The listing builds one solid part. Answer for the finished solid, in the listing's coordinates (mm). A direction names the side the tool comes from. Give positions to 0.01 mm unless a question says otherwise; leave off trailing zeros. Order: outer loops, then holes, each group sorted by start corner. A loop starts at its lowest first (then second) coordinate and runs counter-clockwise, first axis right, second up. Notation, with made-up numbers: (-8, -16) - (7, -16) arc R30 ccw to (7, 20) - close; hole circle Ø9 at (41.5, -1). An arc over 180 degrees is marked (long way). Use a Markdown table: item, result. Add a question column.
1) The mould has two halves that part along Y. Classify faces 5 (the face through (-16.926, 7, 5)), 6 (the face through (-26, -2, 29)), 7 (the face through (-13.66, -9.32, 5.2)), 8 (the face through (-32, 5, 5)): released by +Y, released by -Y, zero draft, split by the parting line, or undercut.
2) Straight lines are drawn through the part: line 1 (Z direction, x = -22.75, y = 5.5); line 2 (Y direction, x = -22, z = 15); line 3 (Y direction, x = -16.25, z = 26). For each, find the intervals that lie inside material, in ascending order.
3) Flat-ended cylindrical pins translate along their axes: pin 1 (1.5 mm diameter, centred on x = -17, z = 13.5, fed in from -Y); pin 2 (3.5 mm diameter, centred on x = -22.93, z = 9.99, fed in from -Y); pin 3 (12 mm diameter, centred on x = -14.5, z = 34.5, fed in from +Y). Find the tip coordinate at first contact, or state that the pin passes through.
4) For faces 1 (the face through (-16.926, -5, 17)), 2 (the face through (-30.926, -5, 21)), 3 (the face through (-16.926, -17, 5)), 4 (the face through (-23, -1, 20.744)), determine the directions among +Z, -Z, +X, -X, +Y, -Y from which every point of the face is accessible in a straight line to the end or side of a thin tool.
5) Find section D-D, the plane x = -19. Determine the outline of the cut face in (y, z).
6) Find section B-B, the plane x = -13. Determine the outline of the cut face in (y, z), plus the area to 3 significant figures.
7) Find section A-A, the plane y = 4.3. Determine the outline of the cut face in (x, z), plus the area to 3 significant figures.
8) Find section C-C, the plane y = -17. Determine the outline of the cut face in (x, z), plus the area to 3 significant figures.
from build123d import *

# Parameters (mm, degrees)
F0_R          = 1.3
F1_DEPTH      = 2
F2_W          = 12
F2_H          = 3
F3_DEPTH      = 18
F3_DEPTH_BACK = 12
F4_W          = 5
F4_H          = 3
F4_W_2        = 2
F4_H_2        = 35.8160760757
F5_DEPTH      = 2
F6_W          = 2
F6_H          = 35.8160760757
F7_DEPTH      = 2
F9_DEPTH      = 5
F11_DEPTH     = 5
F12_R         = 1
F13_DEPTH     = 5
F14_W         = 2.25
F14_H         = 11.5
F15_DEPTH     = 3
F16_R         = 1.2
F17_DEPTH     = 3
F19_DEPTH     = 2


with BuildPart() as f1:
    # F0 (on Front) → F1 (new body)
    with BuildSketch(Plane.XZ):
        with BuildLine():
            Line((-16.9256870747, 6.6775220651), (-16.9256870747, 9.9935981408))
            Line((-16.9256870747, 9.9935981408), (-16.9256870747, 10.6775220651))
            Line((-16.9256870747, 10.6775220651), (-16.9256870747, 42.4935981408))
            ThreePointArc((-16.9256870747, 42.4935981408), (-22.9256870747, 48.4935981408), (-28.9256870747, 42.4935981408))
            Line((-28.9256870747, 42.4935981408), (-28.9256870747, 9.9935981408))
            Line((-28.9256870747, 9.9935981408), (-28.9256870747, 6.6775220651))
            Line((-28.9256870747, 6.6775220651), (-16.9424954802, 6.6775220651))
            Line((-16.9424954802, 6.6775220651), (-16.9256870747, 6.6775220651))
        make_face()
        with Locations((-22.9256870747, 9.9935981408)):
            Circle(F0_R, mode=Mode.SUBTRACT)
        with Locations((-22.9256870747, 42.4935981408)):
            Circle(F0_R, mode=Mode.SUBTRACT)
    extrude(amount=F1_DEPTH)

    # F2 (on face) → F3 (join, two sides)
    with BuildSketch(Plane.XZ.offset(2)) as f3_sk:
        with Locations((-22.9256870747, 5.1775220651)):
            Rectangle(F2_W, F2_H)
    extrude(amount=F3_DEPTH)
    extrude(f3_sk.sketch, amount=-F3_DEPTH_BACK)

    # F4 (on face) → F5 (join)
    with BuildSketch(Plane.YZ.offset(-16.9256870747)):
        Polygon((-13, 6.6775220651), (-2, 6.6775220651), (-2, 42.4935981408), align=None)
        Polygon((0, 3.6775220651), (0, 6.6775220651), (-2, 6.6775220651), (-13, 6.6775220651), (-13, 3.6775220651), align=None)
        with Locations((2.5, 5.1775220651)):
            Rectangle(F4_W, F4_H)
        with Locations((-1, 24.5855601029)):
            Rectangle(F4_W_2, F4_H_2)
    extrude(amount=F5_DEPTH)

    # F6 (on face) → F7 (join)
    with BuildSketch(Plane(origin=(-28.9256870747, 0, 0), x_dir=(0, -1, 0), z_dir=(-1, 0, 0))):
        Polygon((0, 6.6775220651), (-5, 6.6775220651), (-5, 3.6775220651), (13, 3.6775220651), (13, 6.6775220651), (2, 6.6775220651), align=None)
        Polygon((2, 42.4935981408), (2, 6.6775220651), (13, 6.6775220651), align=None)
        with Locations((1, 24.5855601029)):
            Rectangle(F6_W, F6_H)
    extrude(amount=F7_DEPTH)

    # F8 (on face) → F9 (join)
    with BuildSketch(Plane(origin=(-30.9256870747, 0, 0), x_dir=(0, -1, 0), z_dir=(-1, 0, 0))):
        Polygon((0, 6.6775220651), (-5, 6.6775220651), (-5, 3.6775220651), (13, 3.6775220651), (13, 6.6775220651), align=None)
    extrude(amount=F9_DEPTH)

    # F10 (on face) → F11 (join)
    with BuildSketch(Plane.YZ.offset(-14.9256870747)):
        Polygon((0, 6.6775220651), (-13, 6.6775220651), (-13, 3.6775220651), (5, 3.6775220651), (5, 6.6775220651), align=None)
    extrude(amount=F11_DEPTH)

    # F12 (on face) → F13 (cut)
    with BuildSketch(Plane.XY.offset(6.6775220651)):
        with Locations((-32.9256870747, 2)):
            Circle(F12_R)
        with Locations((-12.9256870747, 2)):
            Circle(F12_R)
        with Locations((-12.9256870747, -10)):
            Circle(F12_R)
        with Locations((-22.9256870747, -5)):
            Circle(F12_R)
        with Locations((-32.9256870747, -10)):
            Circle(F12_R)
        with Locations((-22.9256870747, -17)):
            Circle(F12_R)
    extrude(amount=-F13_DEPTH, mode=Mode.SUBTRACT)

    # F14 (on face) → F15 (cut)
    with BuildSketch(Plane(origin=(0, 0, 0), x_dir=(-1, 0, 0), z_dir=(0, 1, 0))):
        with Locations((24.0506870747, 26.4935981408)):
            Rectangle(F14_W, F14_H)
        with Locations((21.8006870747, 26.4935981408)):
            Rectangle(F14_W, F14_H)
    extrude(amount=-F15_DEPTH, mode=Mode.SUBTRACT)

    # F16 (on face) → F17 (cut)
    with BuildSketch(Plane.XY.offset(6.6775220651)):
        with Locations((-18.7256870747, 4.3)):
            Circle(F16_R)
    extrude(amount=-F17_DEPTH, mode=Mode.SUBTRACT)

    # F18 (on face) → F19 (join)
    with BuildSketch(Plane(origin=(0, 0, 0), x_dir=(-1, 0, 0), z_dir=(0, 1, 0))):
        with BuildLine():
            Line((28.9256870747, 42.4935981408), (30.9256870747, 42.4935981408))
            ThreePointArc((30.9256870747, 42.4935981408), (22.9256870747, 50.4935981408), (14.9256870747, 42.4935981408))
            Line((14.9256870747, 42.4935981408), (16.9256870747, 42.4935981408))
            ThreePointArc((16.9256870747, 42.4935981408), (22.9256870747, 48.4935981408), (28.9256870747, 42.4935981408))
        make_face()
    extrude(amount=-F19_DEPTH)


solid = f1.part
The answers:
| question | item | result |
|---|---|---|
| 1 | face 5 | zero draft |
| 1 | face 6 | released by -Y |
| 1 | face 7 | undercut |
| 1 | face 8 | released by +Y |
| 2 | line 1 | 3.68 to 6.68 |
| 2 | line 2 | -2 to 0 |
| 2 | line 3 | -7.07 to 0 |
| 3 | pin 1 | y = -11.13 |
| 3 | pin 2 | y = -2 |
| 3 | pin 3 | y = 0 |
| 4 | face 1 | +Z, -Y |
| 4 | face 2 | +Z, -X, +Y, -Y |
| 4 | face 3 | +Z, -Z, +X, -Y |
| 4 | face 4 | +Y, -Y |
| 5 | outline | (-20, 3.68) - (3.13, 3.68) - (3.13, 6.68) - (0, 6.68) - (0, 49.46) - (-2, 49.46) - (-2, 6.68) - (-20, 6.68) - close; (5.47, 3.68) - (10, 3.68) - (10, 6.68) - (5.47, 6.68) - close |
| 6 | outline | (-13, 3.68) - (-11, 3.68) - (-11, 6.68) - (-13, 6.68) - close; (-9, 3.68) - (1, 3.68) - (1, 6.68) - (-9, 6.68) - close; (3, 3.68) - (5, 3.68) - (5, 6.68) - (3, 6.68) - close |
| 6 | area | 42.0 mm2 |
| 7 | outline | (-35.93, 3.68) - (-19.93, 3.68) - (-19.93, 6.68) - (-35.93, 6.68) - close; (-17.53, 3.68) - (-9.93, 3.68) - (-9.93, 6.68) - (-17.53, 6.68) - close |
| 7 | area | 70.8 mm2 |
| 8 | outline | (-28.93, 3.68) - (-23.93, 3.68) - (-23.93, 6.68) - (-28.93, 6.68) - close; (-21.93, 3.68) - (-16.93, 3.68) - (-16.93, 6.68) - (-21.93, 6.68) - close |
| 8 | area | 30.0 mm2 |
